Autodesk Fusion 360 part; units mm, degrees
sketch "Sketch1" plane through (0, 0, 0) normal (1, 0, 0) x (0, 0, -1)
  circle A0 centre (0, 0) radius 28.5
  dimension "d1" = 57
extrude "Extrude1" add sketch "Sketch1" along normal blind 15
sketch "Sketch2" plane through (0, 0, 0) normal (1, 0, 0) x (0, 0, -1)
  circle A0 centre (0, 0) radius 27.5
  dimension "d4" = 55
extrude "Extrude2" add sketch "Sketch2" against normal blind 55
sketch "Sketch3" plane through (-55, 0, 0) normal (-1, 0, 0) x (0, 0, 1)
  circle A0 centre (0, 0) radius 27.5
  circle A1 centre (0, 0) radius 28.5
extrude "Extrude3" add sketch "Sketch3" along normal blind 5 contours A0 | A1
sketch "Sketch4" plane through (-60, 0, 0) normal (-1, 0, 0) x (0, 0, 1)
  circle A0 centre (0, 0) radius 28.5
  circle A1 centre (0, 0) radius 28.5
extrude "Extrude4" add sketch "Sketch4" along normal blind 45
sketch "Sketch5" plane through (-105, 0, 0) normal (-1, 0, 0) x (0, 0, 1)
  circle A0 centre (0, 0) radius 28.5
  circle A1 centre (0, 0) radius 15.9875
  dimension "d11" = 31.975
extrude "Extrude5" add sketch "Sketch5" along normal blind 2 contours A1
sketch "Sketch6" plane through (-107, 0, 0) normal (-1, 0, 0) x (0, 0, 1)
  circle A0 centre (0, 0) radius 15.9875
  circle A1 centre (0, 0) radius 5.9925
  dimension "d14" = 11.985
extrude "Extrude6" add sketch "Sketch6" along normal blind 20 contours A1
sketch "Sketch7" plane through (-127, 0, 0) normal (-1, 0, 0) x (0, 0, 1)
  circle A0 centre (0, 0) radius 5.9925
  circle A1 centre (0, 0) radius 2
  dimension "d17" = 4
extrude "Extrude7" cut sketch "Sketch7" against normal blind 15 contours A1
equation "d11 = 32 mm - 0.025 mm"
equation "d14 = 12 mm - 0.015 mm"
Read the model definition and answer for the solid it produces. Units are mm, in the model's axes. A direction names the side the tool comes from. Round coordinates to 2 decimals unless told otherwise and drop trailing zeros. Write each loop counter-clockwise with the first axis right and the second up, starting at its lowest first coordinate (ties: lowest second). Pieces come first, ordered by that corner, then holes. Notation, with made-up numbers: (44, 41) - (71, 41) arc R16 cw to (71, 64) - close; hole circle Ø3 at (20, -35). An arc over 180 degrees is marked (long way). Use CSV: the item, a comma, the result in double quotes.
Q1. Straight lines are drawn through the part: line 1 along Y through (x, z) = (-120, 0); line 2 along X through (y, z) = (-13, -4.5); line 3 along X through (y, z) = (25.5, 5). For each, find the intervals that lie inside material, in ascending order.
Values:
line 1,"y = -5.99 to -2, 2 to 5.99"
line 2,"x = -107 to 15"
line 3,"x = -105 to 15"
Q2. Find section D-D, the plane y = -18.5. Write down the section's boundary in (x, z), then the cut area to 3 significant figures.
Values:
outline,"(-105, -21.68) - (-55, -21.68) - (-55, -20.35) - (0, -20.35) - (0, -21.68) - (15, -21.68) - (15, 21.68) - (0, 21.68) - (0, 20.35) - (-55, 20.35) - (-55, 21.68) - (-105, 21.68) - close"
area,"5,060 mm²"
Q3. Find section B-B, the plane z = 11.5. Write down the section's boundary in (x, y).
Values:
outline,"(-107, -11.11) - (-105, -11.11) - (-105, -26.08) - (-55, -26.08) - (-55, -24.98) - (0, -24.98) - (0, -26.08) - (15, -26.08) - (15, 26.08) - (0, 26.08) - (0, 24.98) - (-55, 24.98) - (-55, 26.08) - (-105, 26.08) - (-105, 11.11) - (-107, 11.11) - close"
Q4. A tool of negligible diameter and unlimited length cuts with its end or side. For faces 1 (the flat face through (15, 0, 0)), 2 (the cylindrical face through (-116.86, 5.85, -1.3)), 3 (the flat face through (-55, 23.4, -14.9)), from which of +Z, -Z, +X, -X, +Y, -Y can it reach the whole face along a straight path? Write none if from no direction.
Values:
face 1,"+Z, -Z, +X, +Y, -Y"
face 2,"-X"
face 3,"none"
Q5. Find section A-A, the plane y = 0. Write down the section's boundary in (x, z).
Values:
outline,"(-127, -5.99) - (-107, -5.99) - (-107, -15.99) - (-105, -15.99) - (-105, -28.5) - (-55, -28.5) - (-55, -27.5) - (0, -27.5) - (0, -28.5) - (15, -28.5) - (15, 28.5) - (0, 28.5) - (0, 27.5) - (-55, 27.5) - (-55, 28.5) - (-105, 28.5) - (-105, 15.99) - (-107, 15.99) - (-107, 5.99) - (-127, 5.99) - (-127, 2) - (-112, 2) - (-112, -2) - (-127, -2) - close"
Q6. Each of these flat-tipped pins is pushed along its axis until it touches: pin 1 Ø6 at (x, y) = (-84, 15.5) entering from +Z; pin 2 Ø12 at (x, z) = (-105.5, 21.5) entering from -Y; pin 3 Ø4 at (x, y) = (-59.5, 21.5) entering from -Z; pin 4 Ø4.5 at (y, z) = (0.5, 0) entering from -X. Where does it stop, or does it pass through?
Values:
pin 1,"stops at z = 25.61"
pin 2,"stops at y = -23.9"
pin 3,"stops at z = -20.78"
pin 4,"stops at x = -127"
Q7. Find section C-C, the plane x = 2. Write down the section's boundary in (y, z).
Values:
outline,"circle Ø57 at (0, 0)"
Q8. Determine the mould class of faces 4 (the cylindrical face through (-120, -2, 0)), 5 (the cylindrical face through (7.395, 10.916, -26.327)), 6 (the flat face through (-112, 0, 0)), 7 (the flat face through (-107, -7, 0)) for opening direction Y: +Y half, -Y half, draft (parallel to the pull), parting line (faces both ways), or undercut.
Values:
face 4,"undercut"
face 5,"parting line"
face 6,"undercut"
face 7,"draft"
